Part model, mm, in its own coordinate system. A direction names the side the tool comes from. Coordinates: 2 decimals unless noted, no trailing zeros. Loops run counter-clockwise (first coordinate to the right, second up) from the corner with the lowest first, then second, coordinate; pieces in that order, holes last. Notation, with made-up numbers: M 5,-22 L 22,-22 A18 cw 22,-12 Z; hole C -1,69.5 d4. An arc over 180 degrees is marked long. Answer as a JSON object with one key per item and string values. Group by question number.
1. Drill centre lines: L1, parallel to Y at x = -52.5, z = 4.45; L2, parallel to X at y = -34.5, z = 2.55; L3, parallel to X at y = -27, z = 3.35. Where is each one in solid material? Low to high.
2. Saw through at A-A on y = 62.5. Write the cut outline in (x, z), then the cut area to 3 significant figures.
3. Saw through at C-C on z = 5.05. Write the cut outline in (x, y).
4. Mould opens along Y. For faces 3 (the face through (-59.1, 70.64, 2.96)), 4 (the face through (-60, 15, 3)), 5 (the face through (54.58, -38.99, 2.96)) say: released by +Y, released by -Y, zero draft, split by the parting line, or undercut.
5. Saw through at D-D on x = 8. Write the cut outline in (y, z), then the cut area to 3 significant figures.
6. 3-axis set-ups, long thin cutter, end or side, ignore diameter. For faces 1 (the face through (-44.14, 54.1, 2.96)), 2 (the face through (-53, -42.5, 3)): which of +Z, -Z, +X, -X, +Y, -Y reach the whole face in a straight line?
7. Saw through at B-B on x = 52.5. Write the cut outline in (y, z).
8. Drop a flat-ended pin along its axis: pin 1 Ø3 at (x, y) = (8, 62.5) entering from +Z. Give the stop position or say it passes through.
from build123d import *

# Parameters (mm, degrees)
SKETCH1_R           = 2
SKETCH1_R_2         = 4.5
BOSS_EXTRUDE1_DEPTH = 6


with BuildPart() as part:
    # Sketch1 → Boss-Extrude1 (new body)
    with BuildSketch(Plane.XY):
        with BuildLine():
            Line((-45, -39.5), (-45, 52))
            ThreePointArc((-45, 52), (-44.121320344, 54.121320344), (-42, 55))
            Line((-42, 55), (42, 55))
            ThreePointArc((42, 55), (44.121320344, 54.121320344), (45, 52))
            Line((45, 52), (45, -39.5))
            ThreePointArc((45, -39.5), (45.878679656, -41.621320344), (48, -42.5))
            Line((48, -42.5), (57, -42.5))
            ThreePointArc((57, -42.5), (59.121320344, -41.621320344), (60, -39.5))
            Line((60, -39.5), (60, 68.5))
            ThreePointArc((60, 68.5), (59.121320344, 70.621320344), (57, 71.5))
            Line((57, 71.5), (-57, 71.5))
            ThreePointArc((-57, 71.5), (-59.121320344, 70.621320344), (-60, 68.5))
            Line((-60, 68.5), (-60, -39.5))
            ThreePointArc((-60, -39.5), (-59.121320344, -41.621320344), (-57, -42.5))
            Line((-57, -42.5), (-48, -42.5))
            ThreePointArc((-48, -42.5), (-45.878679656, -41.621320344), (-45, -39.5))
        make_face()
        with Locations((8, 62.5)):
            Circle(SKETCH1_R, mode=Mode.SUBTRACT)
        with Locations((-8, 62.5)):
            Circle(SKETCH1_R, mode=Mode.SUBTRACT)
        with Locations((-52.5, -35)):
            Circle(SKETCH1_R_2, mode=Mode.SUBTRACT)
        with Locations((52.5, -35)):
            Circle(SKETCH1_R_2, mode=Mode.SUBTRACT)
        with Locations((-52.5, 0)):
            Circle(SKETCH1_R_2, mode=Mode.SUBTRACT)
        with Locations((52.5, 0)):
            Circle(SKETCH1_R_2, mode=Mode.SUBTRACT)
    extrude(amount=BOSS_EXTRUDE1_DEPTH)


solid = part.part
Outcome:
{
 "1": {"L1": "y = -42.5 to -39.5, -30.5 to -4.5, 4.5 to 71.5", "L2": "x = -60 to -56.97, -48.03 to -45, 45 to 48.03, 56.97 to 60", "L3": "x = -60 to -45, 45 to 60"},
 "2": {"outline": "M -60,0 L -10,0 L -10,6 L -60,6 Z; M -6,0 L 6,0 L 6,6 L -6,6 Z; M 10,0 L 60,0 L 60,6 L 10,6 Z", "area": "672 mm²"},
 "3": {"outline": "M -60,-39.5 A3 ccw -57,-42.5 L -48,-42.5 A3 ccw -45,-39.5 L -45,52 A3 cw -42,55 L 42,55 A3 cw 45,52 L 45,-39.5 A3 ccw 48,-42.5 L 57,-42.5 A3 ccw 60,-39.5 L 60,68.5 A3 ccw 57,71.5 L -57,71.5 A3 ccw -60,68.5 Z; hole C -52.5,-35 d9; hole C -52.5,0 d9; hole C -8,62.5 d4; hole C 8,62.5 d4; hole C 52.5,-35 d9; hole C 52.5,0 d9"},
 "4": {"face 3": "released by +Y", "face 4": "zero draft", "face 5": "undercut"},
 "5": {"outline": "M 55,0 L 60.5,0 L 60.5,6 L 55,6 Z; M 64.5,0 L 71.5,0 L 71.5,6 L 64.5,6 Z", "area": "75.0 mm²"},
 "6": {"face 1": "+Z, -Z, -Y", "face 2": "+Z, -Z, +X, -X, -Y"},
 "7": {"outline": "M -42.5,0 L -39.5,0 L -39.5,6 L -42.5,6 Z; M -30.5,0 L -4.5,0 L -4.5,6 L -30.5,6 Z; M 4.5,0 L 71.5,0 L 71.5,6 L 4.5,6 Z"},
 "8": {"pin 1": "passes through"}
}
